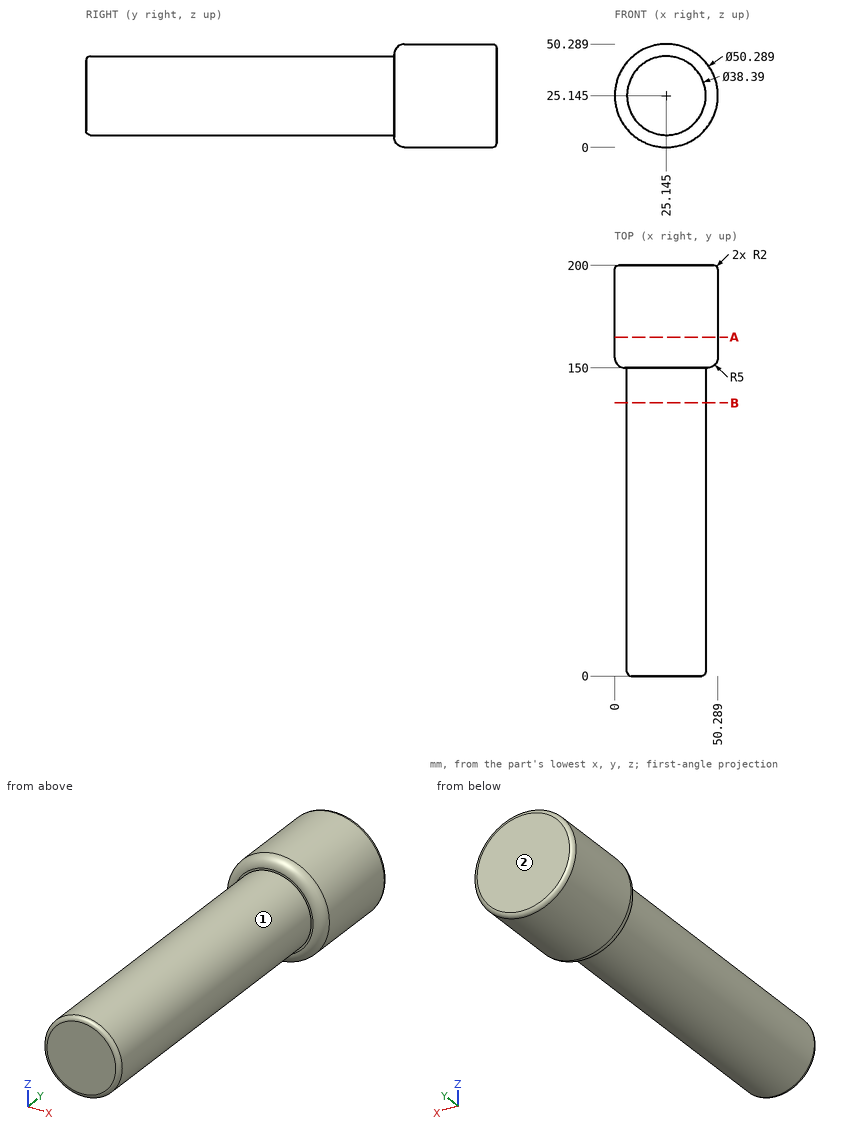
Study the drawing (mm; zero at the part's minimum x, y, z) and answer. A direction names the side the tool comes from. Coordinates: 2 decimals unless noted, no trailing zeros. Write each loop counter-clockwise with the first axis right and the second up, starting at its lowest first coordinate (ties: lowest second). Pieces come first, ordered by that corner, then holes.
Q1. Find the intervals of material crossed by line 1 (X direction, y = 78, z = 25); line 2 (Y direction, x = 33, z = 43.5); line 3 (Y direction, x = 13.5, z = 38) (1 decimal), in increasing order.
Q2. A cutting plane is placed at A-A, the plane y = 165. Give the vertices of the cut face in (x, z) (1 decimal).
Q3. Each of these flat-tipped pins is pushed along its axis until it touches: pin 1 Ø10 at (x, y) = (30, 66.5) entering from -Z; pin 2 Ø8 at (y, z) = (124.5, 11) entering from -X; pin 3 Ø8 at (y, z) = (157, 13.5) entering from -X. Where does it stop, or does it pass through?
Q4. A cutting plane is placed at B-B, the plane y = 133. Give the vertices of the cut face in (x, z) (1 decimal).
Q5. Which of the six approach directions +Z, -Z, +X, -X, +Y, -Y give full straight-line access (tool end or side, diameter ignored) to the marked faces 1 and 2?
Findings below:
1. line 1: x = 5.95 to 44.34
1. line 2: y = 150 to 200
1. line 3: y = 0 to 200
2. outline: circle Ø50.3 at (25.1, 25.1)
3. pin 1: stops at z = 5.95
3. pin 2: stops at x = 8.85
3. pin 3: stops at x = 1.19
4. outline: circle Ø38.4 at (25.1, 25.1)
5. face 1: -Y
5. face 2: +Z, -Z, +X, -X, +Y
